from build123d import *

# Parameters (mm, degrees)
SKETCH1_W           = 46.2
SKETCH1_H           = 18.6
BOSS_EXTRUDE1_DEPTH = 3.4
CUT_EXTRUDE1_DEPTH  = 42.2
SKETCH3_W           = 14.6
SKETCH3_H           = 14.6
CUT_EXTRUDE2_DEPTH  = 26.132847033
FILLET1_R           = 0.5


with BuildPart() as part:
    # Sketch1 → Boss-Extrude1 (new body)
    with BuildSketch(Plane(origin=(0, 0, 0), x_dir=(1, 0, 0), z_dir=(0, 1, 0))):
        Rectangle(SKETCH1_W, SKETCH1_H)
    extrude(amount=BOSS_EXTRUDE1_DEPTH)

    # Sketch2 → Cut-Extrude1 (cut)
    with BuildSketch(Plane(origin=(23.1, 0, 0), x_dir=(0, 0, -1), z_dir=(1, 0, 0))):
        Polygon((2, 3.4), (-2, 3.4), (-3.962990915, 0), (3.962990915, 0), align=None)
    extrude(amount=-CUT_EXTRUDE1_DEPTH, mode=Mode.SUBTRACT)

    # Sketch3 → Cut-Extrude2 (cut, through all)
    with BuildSketch(Plane(origin=(0, 3.4, 0), x_dir=(1, 0, 0), z_dir=(0, 1, 0))):
        with Locations((11.8, 0)):
            Rectangle(SKETCH3_W, SKETCH3_H)
    extrude(amount=-CUT_EXTRUDE2_DEPTH, mode=Mode.SUBTRACT)

    # Fillet1
    fillet1_edges = [part.edges().sort_by_distance(p)[0] for p in [
        (-7.3, 3.4, 2),
        (-7.3, 3.4, -2),
        (21.1, 3.4, -2),
        (21.1, 3.4, 2),
    ]]
    fillet(fillet1_edges, radius=FILLET1_R)


solid = part.part
Design review of the part built by this model. Coordinates are the model's own, in mm. A direction names the side the tool comes from. Round coordinates to 2 decimals unless told otherwise and drop trailing zeros. Loops run counter-clockwise (first coordinate to the right, second up) from the corner with the lowest first, then second, coordinate; pieces in that order, holes last. Notation, with made-up numbers: M 36,31.5 L 90,31.5 A13 cw 90,53.5 Z; hole C 25,-16 d3. An arc over 180 degrees is marked long. Answer as a JSON object with one key per item and string values.
Item 1: We need section C-C on y = 1.9. Give the boundary of the cut face in (x, z).
Answer sheet:
{"outline": "M -23.1,-9.3 L 23.1,-9.3 L 23.1,-2.87 L 19.1,-2.87 L 19.1,-7.3 L 4.5,-7.3 L 4.5,-2.87 L -19.1,-2.87 L -19.1,2.87 L 4.5,2.87 L 4.5,7.3 L 19.1,7.3 L 19.1,2.87 L 23.1,2.87 L 23.1,9.3 L -23.1,9.3 Z"}
Item 2: The part is to be moulded in two halves that separate along X. For faces 1 (the flat face through (21.128, 1.306, -3.209)), 2 (the flat face through (19.1, 2, 5)), 3 (the flat face through (-23.1, 2, 0)), say which applies: pulls with the +X half, pulls with the -X half, needs draft (parallel to the pull), parting line crosses it, or undercut.
Answer sheet:
{"face 1": "needs draft", "face 2": "undercut", "face 3": "pulls with the -X half"}
Item 3: We need section B-B on z = 6. Give the boundary of the cut face in (x, y).
Answer sheet:
{"outline": "M -23.1,0 L 4.5,0 L 4.5,3.4 L -23.1,3.4 Z; M 19.1,0 L 23.1,0 L 23.1,3.4 L 19.1,3.4 Z"}
Item 4: We need section A-A on x = 6.5. Give the boundary of the cut face in (y, z), and give its area (3 significant figures).
Answer sheet:
{"outline": "M 0,-9.3 L 3.4,-9.3 L 3.4,-7.3 L 0,-7.3 Z; M 0,7.3 L 3.4,7.3 L 3.4,9.3 L 0,9.3 Z", "area": "13.6 mm^2"}
Item 5: Wall thickness on L1, parallel to X at y = 3.1, z = -7.25; L2, parallel to Z at x = 10, y = 0.9; L3, parallel to X at y = 0.4, z = 3: over which ranges is each line inside the solid? List them lowest first. Write a range as from..to.
Answer sheet:
{"L1": "x = -23.1..4.5, 19.1..23.1", "L2": "z = -9.3..-7.3, 7.3..9.3", "L3": "x = -23.1..-19.1"}
Item 6: Clearance check with flat-ended pins moving along their axes: P1, Ø1, axis at y = 1, z = -1, coming from the +X side; P2, Ø1, axis at x = -13, z = -3, coming from the -Y side. State where each tip first meets the part, or that it passes through.
Answer sheet:
{"P1": "stops at x = -19.1", "P2": "stops at y = 0.8"}
Item 7: We need section D-D on x = -18.5. Give the boundary of the cut face in (y, z).
Answer sheet:
{"outline": "M 0,-9.3 L 3.4,-9.3 L 3.4,-2.87 A0.5 ccw 2.65,-2.43 L 0,-3.96 Z; M 0,3.96 L 2.65,2.43 A0.5 ccw 3.4,2.87 L 3.4,9.3 L 0,9.3 Z"}
Item 8: Machinability: for faces 4 (the flat face through (-5, 3.4, -4)), 5 (the flat face through (21.13, 1.34, 3.19)), 6 (the flat face through (4.5, 2, -5)), which of the approach directions +Z, -Z, +X, -X, +Y, -Y give a long, thin tool a straight path to every point of the face, cutting with its end or side? Answer none if there is none.
Answer sheet:
{"face 4": "+Z, -Z, +X, -X, +Y", "face 5": "+X, -Y", "face 6": "+Y, -Y"}
